from build123d import *

# Parameters (mm, degrees)
SKETCH1_R               = 13
BOSS_EXTRUDE1_DEPTH     = 50
SKETCH6_W               = 5
SKETCH6_H               = 26
BOSS_EXTRUDE3_DEPTH     = 6
BOSS_EXTRUDE4_DEPTH     = 5
CUT_EXTRUDE1_DEPTH      = 54.937463789
CUT_EXTRUDE1_DEPTH_BACK = 54.937463789
SKETCH10_R              = 2.5
SKETCH12_W              = 4.8936145
SKETCH12_H              = 26
CUT_EXTRUDE2_DEPTH      = 18
CUT_EXTRUDE3_DEPTH      = 54.272882407
CUT_EXTRUDE3_DEPTH_BACK = 54.272882407
SKETCH13_R              = 2.5


with BuildPart() as part:
    # Sketch1 → Boss-Extrude1 (new body)
    with BuildSketch(Plane(origin=(0, 0, 0), x_dir=(0, 0, -1), z_dir=(1, 0, 0))):
        Circle(SKETCH1_R)
    extrude(amount=-BOSS_EXTRUDE1_DEPTH)

    # Sketch6 → Boss-Extrude3 (add)
    with BuildSketch(Plane(origin=(0, 0, 0), x_dir=(0, 0, -1), z_dir=(1, 0, 0))):
        Rectangle(SKETCH6_W, SKETCH6_H)
    extrude(amount=BOSS_EXTRUDE3_DEPTH)

    # Sketch8 → Boss-Extrude4 (add)
    with BuildSketch(Plane.XY.offset(2.5)):
        with BuildLine():
            Line((6, 13), (6, -13))
            ThreePointArc((6, -13), (19, 0), (6, 13))
        make_face()
    extrude(amount=-BOSS_EXTRUDE4_DEPTH)

    # Sketch10 → Cut-Extrude1 (cut, two sides: drawn at the far end of the back side and taken through both)
    with BuildSketch(Plane.XY.offset(2.5).offset(-CUT_EXTRUDE1_DEPTH_BACK)):
        with Locations((15.9, -0.5)):
            Circle(SKETCH10_R)
    extrude(amount=CUT_EXTRUDE1_DEPTH + CUT_EXTRUDE1_DEPTH_BACK, mode=Mode.SUBTRACT)

    # Sketch12 → Cut-Extrude2 (cut)
    with BuildSketch(Plane.ZY.offset(50)):
        Rectangle(SKETCH12_W, SKETCH12_H)
    extrude(amount=-CUT_EXTRUDE2_DEPTH, mode=Mode.SUBTRACT)

    # Sketch13 → Cut-Extrude3 (cut, two sides: drawn at the far end of the back side and taken through both)
    with BuildSketch(Plane.XY.offset(-CUT_EXTRUDE3_DEPTH_BACK)):
        with Locations(Location((-45, -0.5, 0), (0, 0, 168.463040967))):
            Circle(SKETCH13_R)
    extrude(amount=CUT_EXTRUDE3_DEPTH + CUT_EXTRUDE3_DEPTH_BACK, mode=Mode.SUBTRACT)


solid = part.part
Can you work these out from the model? Positions are in its coordinate system, mm. A direction names the side the tool comes from. Coordinates: 2 decimals unless noted, no trailing zeros. Order: outer loops, then holes, each group sorted by start corner. A loop starts at its lowest first (then second) coordinate and runs counter-clockwise, first axis right, second up. Notation, with made-up numbers: (-9.5, 28) -> (29.5, 28) arc R19 ccw to (29.5, 64) -> close; hole circle Ø5 at (-4, 86). An arc over 180 degrees is marked (long way). Use one line per item in the form item = value.
Q1. Which directions (+Z, -Z, +X, -X, +Y, -Y) give clear straight access to the entire face, cutting with the end or side of a thin tool? Please do faces 4 (the face through (-50, 0, -6)), 5 (the face through (-42.575, -1.107, 7.65)), 6 (the face through (-41, 0, 2.447)), 7 (the face through (0, 0, -7)), 8 (the face through (0, 0, 7)).
From the geometry:
face_4 = +Z, -Z, -X, +Y, -Y
face_5 = +Z, -Z
face_6 = -X, +Y, -Y
face_7 = -Z, +X, +Y, -Y
face_8 = +Z, +X, +Y, -Y
Q2. Imagine slicing it at D-D, the plane x = -12. List the corners of the cut face in (y, z) for me, then the cut area to 3 significant figures.
From the geometry:
outline = circle Ø26 at (0, 0)
area = 531 mm²
Q3. Imagine slicing it at A-A, the plane y = -2.25. List the corners of the cut face in (x, z) for me.
From the geometry:
outline = (-50, -12.8) -> (-46.79, -12.8) -> (-46.79, -2.45) -> (-50, -2.45) -> close; (-50, 2.45) -> (-46.79, 2.45) -> (-46.79, 12.8) -> (-50, 12.8) -> close; (-43.21, -12.8) -> (0, -12.8) -> (0, -2.5) -> (14.11, -2.5) -> (14.11, 2.5) -> (0, 2.5) -> (0, 12.8) -> (-43.21, 12.8) -> (-43.21, 2.45) -> (-32, 2.45) -> (-32, -2.45) -> (-43.21, -2.45) -> close; (17.69, -2.5) -> (18.8, -2.5) -> (18.8, 2.5) -> (17.69, 2.5) -> close
Q4. Imagine slicing it at C-C, the plane y = -10.75. List the corners of the cut face in (x, z) for me, then the cut area to 3 significant figures.
From the geometry:
outline = (-50, -7.31) -> (0, -7.31) -> (0, -2.5) -> (13.31, -2.5) -> (13.31, 2.5) -> (0, 2.5) -> (0, 7.31) -> (-50, 7.31) -> (-50, 2.45) -> (-32, 2.45) -> (-32, -2.45) -> (-50, -2.45) -> close
area = 709 mm²
Q5. I need wall thicknesses on L1, parallel to X at y = -0.5, z = 1.15; L2, parallel to X at y = -0.5, z = -10; L3, parallel to X at y = 6.75, z = 10. Which ranges of each line are inside material? Lowest first, please.
From the geometry:
L1 = -32 to 13.4, 18.4 to 18.99
L2 = -50 to -47.5, -42.5 to 0
L3 = -50 to 0
Q6. Imagine slicing it at B-B, the plane z = 9.5. List the corners of the cut face in (x, y) for me.
From the geometry:
outline = (-50, -8.87) -> (0, -8.87) -> (0, 8.87) -> (-50, 8.87) -> close; hole circle Ø5 at (-45, -0.5)
Q7. Will these pins go through, and if not, where does the flat tip stop? P1, Ø3, axis at x = 6.5, y = -9, coming from the -Z side; P2, Ø6, axis at x = -21, y = -8.5, coming from the +Z side; P3, Ø11.5, axis at y = -5.5, z = 9, coming from the +X side.
From the geometry:
P1 = -2.5
P2 = 11.78
P3 = 0
Q8. We'd pull the mould along Z, two halves only. Please class faces 1 (the face through (-42.575, -1.107, -7.797)), 2 (the face through (-32, 0, 0)), 3 (the face through (7, 0, 2.5)): released by +Z, released by -Z, zero draft, split by the parting line, or undercut.
From the geometry:
face_1 = zero draft
face_2 = undercut
face_3 = released by +Z
